from build123d import *

# Parameters (mm, degrees)
SCHIZZO1_R                   = 1.5
SCHIZZO1_W                   = 25
SCHIZZO1_H                   = 4
ESTRUSIONE_ESTRUSIONE2_DEPTH = 4


with BuildPart() as part:
    # Schizzo1 → Estrusione-Estrusione2 (new body)
    with BuildSketch(Plane.XY):
        with BuildLine():
            Line((-22.627416998, -7.5), (0, -7.5))
            ThreePointArc((0, -7.5), (6.929096494, -2.870125743), (5.303300859, 5.303300859))
            Line((5.303300859, 5.303300859), (-17.324116139, 27.930717857))
            ThreePointArc((-17.324116139, 27.930717857), (-23.686333927, 30.052287026), (-29.20181593, 26.236749163))
            Line((-29.20181593, 26.236749163), (-45.934294533, 4.586300077))
            ThreePointArc((-45.934294533, 4.586300077), (-46.732282324, -3.305506726), (-40, -7.5))
            Line((-40, -7.5), (-22.627416998, -7.5))
        make_face()
        Circle(SCHIZZO1_R, mode=Mode.SUBTRACT)
        with Locations((-22.627416998, 22.627416998)):
            Circle(SCHIZZO1_R, mode=Mode.SUBTRACT)
        with Locations((-40, 0)):
            Circle(SCHIZZO1_R, mode=Mode.SUBTRACT)
        with Locations((-22.5, -2.5)):
            Rectangle(SCHIZZO1_W, SCHIZZO1_H, mode=Mode.SUBTRACT)
    extrude(amount=ESTRUSIONE_ESTRUSIONE2_DEPTH)


solid = part.part
Geometry: final body of the model. Coordinates: model frame, mm. A direction names the side the tool comes from. Coordinates: 2 decimals unless noted, no trailing zeros. Order: outer loops, then holes, each group sorted by start corner. A loop starts at its lowest first (then second) coordinate and runs counter-clockwise, first axis right, second up.
1) Ray query, probe 1 along X at (y, z) = (-1, 3.2); probe 2 along Y at (x, z) = (0, 1.55); probe 3 along Y at (x, z) = (-14.5, 0.45). Return the intervals inside material, ascending.
Result sheet:
probe 1: x = -47.43 to -41.12, -38.88 to -35, -10 to -1.12, 1.12 to 7.43
probe 2: y = -7.5 to -1.5, 1.5 to 10.61
probe 3: y = -7.5 to -4.5, -0.5 to 25.11
2) Section C-C (y = 9). Return loops of the section in (x, z).
Result sheet:
outline: (-42.52, 0) - (1.61, 0) - (1.61, 4) - (-42.52, 4) - close
3) Draft query along Y for faces 1 (the flat face through (-20, 7, 0)), 2 (the flat face through (-10, -3, 2)), 3 (the cylindrical face through (6.881, -2.984, 1.972)). Return one class per face: released by +Y, released by -Y, zero draft, split by the parting line, or undercut.
Result sheet:
face 1: zero draft
face 2: undercut
face 3: split by the parting line
4) Set-up query: faces 4 (the cylindrical face through (-24, 30, 2)), 5 (the flat face through (-23, -0.5, 2)). Return all of +Z, -Z, +X, -X, +Y, -Y with unobstructed straight access to the full face (end or side cutting, diameter ignored); none if empty.
Result sheet:
face 4: +Z, -Z, +Y
face 5: +Z, -Z
5) Section D-D (x = -7). Return loops of the section in (y, z).
Result sheet:
outline: (-7.5, 0) - (17.61, 0) - (17.61, 4) - (-7.5, 4) - close
6) Section B-B (z = 2.9). Return loops of the section in (x, y), then the cut area to 3 significant figures.
Result sheet:
outline: (-45.93, 4.59) arc R7.5 ccw to (-40, -7.5) - (0, -7.5) arc R7.5 ccw to (5.3, 5.3) - (-17.32, 27.93) arc R7.5 ccw to (-29.2, 26.24) - close; hole circle Ø3 at (-40, 0); hole (-35, -4.5) - (-10, -4.5) - (-10, -0.5) - (-35, -0.5) - close; hole circle Ø3 at (-22.63, 22.63); hole circle Ø3 at (0, 0)
area: 1,260 mm2
7) First-contact query: P1, Ø2, axis at y = 23.5, z = 3, coming from the -X side; P2, Ø1, axis at y = -1.5, z = 3.5, coming from the +X side; P3, Ø1.5, axis at x = -40, y = 14.5, coming from the +Z side; P4, Ø2, axis at y = -2.5, z = 2, coming from the +X side. Flat tips, straight axial feed; report the tip coordinate or a pass-through.
Result sheet:
P1: stops at x = -32.09
P2: stops at x = 7.43
P3: passes through
P4: stops at x = 7.35
8) Section A-A (x = -16.5). Return loops of the section in (y, z).
Result sheet:
outline: (-7.5, 0) - (-4.5, 0) - (-4.5, 4) - (-7.5, 4) - close; (-0.5, 0) - (27.11, 0) - (27.11, 4) - (-0.5, 4) - close
